```python
from build123d import *

# Parameters (mm, degrees)
SKETCH1_R           = 6.35
BOSS_EXTRUDE1_DEPTH = 3.175
FILLET1_R           = 2
FILLET2_R           = 10
FILLET3_R           = 20


with BuildPart() as part:
    # Sketch1 → Boss-Extrude1 (new, symmetric)
    with BuildSketch(Plane.XY):
        Polygon((75.336239509, 30), (-75.336239509, 30), (-95.474630657, 6), (-95.474630657, -6), (-75.336239509, -30), (75.336239509, -30), (95.474630657, -6), (95.474630657, 6), align=None)
        with BuildLine():
            Line((-88.474630657, -1.3375), (-88.474630657, 1.3375))
            ThreePointArc((-88.474630657, 1.3375), (-88.714791341, 1.656946712), (-88.341203698, 1.798917233))
            ThreePointArc((-88.341203698, 1.798917233), (-82.55, 0), (-88.341203698, -1.798917233))
            ThreePointArc((-88.341203698, -1.798917233), (-88.714791341, -1.656946712), (-88.474630657, -1.3375))
        make_face(mode=Mode.SUBTRACT)
        with Locations((-51.435, 0)):
            Circle(SKETCH1_R, mode=Mode.SUBTRACT)
        with Locations((-17.145, 0)):
            Circle(SKETCH1_R, mode=Mode.SUBTRACT)
        with Locations((17.145, 0)):
            Circle(SKETCH1_R, mode=Mode.SUBTRACT)
        with Locations((51.435, 0)):
            Circle(SKETCH1_R, mode=Mode.SUBTRACT)
        with BuildLine():
            ThreePointArc((88.341203698, 1.798917233), (88.714791341, 1.656946712), (88.474630657, 1.3375))
            Line((88.474630657, 1.3375), (88.474630657, -1.3375))
            ThreePointArc((88.474630657, -1.3375), (88.714791341, -1.656946712), (88.341203698, -1.798917233))
            ThreePointArc((88.341203698, -1.798917233), (82.55, 0), (88.341203698, 1.798917233))
        make_face(mode=Mode.SUBTRACT)
    extrude(amount=BOSS_EXTRUDE1_DEPTH, both=True)

    # Fillet1
    fillet1_edges = [part.edges().sort_by_distance(p)[0] for p in [
        (-88.341203698, 1.798917233, 0),
        (-88.474630657, 1.3375, 0),
        (-88.474630657, -1.3375, 0),
        (-88.341203698, -1.798917233, 0),
        (88.341203698, -1.798917233, 0),
        (88.474630657, -1.3375, 0),
        (88.474630657, 1.3375, 0),
        (88.341203698, 1.798917233, 0),
    ]]
    fillet(fillet1_edges, radius=FILLET1_R)

    # Fillet2
    fillet2_edges = [part.edges().sort_by_distance(p)[0] for p in [
        (95.474630657, 6, 0),
        (95.474630657, -6, 0),
        (-95.474630657, -6, 0),
        (-95.474630657, 6, 0),
    ]]
    fillet(fillet2_edges, radius=FILLET2_R)

    # Fillet3
    fillet3_edges = [part.edges().sort_by_distance(p)[0] for p in [
        (75.336239509, -30, 0),
        (-75.336239509, -30, 0),
        (-75.336239509, 30, 0),
        (75.336239509, 30, 0),
    ]]
    fillet(fillet3_edges, radius=FILLET3_R)


solid = part.part
```
Check sheet for the modelled part. Datum: model origin and axes. Units: mm. Round coordinates to 2 decimals unless told otherwise and drop trailing zeros. Write each loop counter-clockwise with the first axis right and the second up, starting at its lowest first coordinate (ties: lowest second). Pieces come first, ordered by that corner, then holes. Notation, with made-up numbers: (7.25, 51) -> (54.25, 51) arc R33 cw to (54.25, 89) -> close; hole circle Ø10 at (5, 48.25). An arc over 180 degrees is marked (long way). One line per question, with ' | ' between items. Start each with the question number.
1. Sectioned sample at A-A, the plane x = -18. Record the cut outline in (y, z) (3 decimals), then the cut area to 3 significant figures.
2. Depth check by flat-ended pin: pin 1 (1.5 mm diameter, centred on y = 4, z = 1, fed in from -X) (3 decimals); pin 2 (1 mm diameter, centred on y = -4.5, z = 0.5, fed in from +X). Enter the tip coordinate at first touch or a pass-through.
3. Scan lines: line 1 along X through (y, z) = (5, -2.5); line 2 along X through (y, z) = (-7, 1.5); line 3 along Y through (x, z) = (-18.5, -2). Record each from-to range of solid material in increasing order. Write a range as from..to.
4. Release check for a two-part mould opening along Y. For faces 1 (the face through (-95.475, 0, 0)), 2 (the face through (94.855, 5.826, -0.044)), 3 (the face through (-45.38, 1.91, -0.04)) record: +Y half, -Y half, draft (parallel to the pull), parting line (faces both ways), or undercut.
5. Sectioned sample at D-D, the plane x = 79.5. Record the cut outline in (y, z) (3 decimals).
6. Sectioned sample at B-B, the plane z = 2. Count the separate pieces of the cut face and the enclosed holes in it, then the cut area to 3 significant figures.
7. Sectioned sample at C-C, the plane x = -54. Record the cut outline in (y, z) (3 decimals), then the cut area to 3 significant figures.
Taken from the geometry:
1) outline: (-30, -3.175) -> (-6.292, -3.175) -> (-6.292, 3.175) -> (-30, 3.175) -> close; (6.292, -3.175) -> (30, -3.175) -> (30, 3.175) -> (6.292, 3.175) -> close | area: 301 mm^2
2) pin 1: stops at x = -95.435 | pin 2: stops at x = 95.34
3) line 1: x = -95.12..-55.35, -47.52..-21.06, -13.23..13.23, 21.06..47.52, 55.35..95.12 | line 2: x = -94.33..94.33 | line 3: y = -30..-6.2, 6.2..30
4) face 1: draft | face 2: +Y half | face 3: undercut
5) outline: (-24.766, -3.175) -> (24.766, -3.175) -> (24.766, 3.175) -> (-24.766, 3.175) -> close
6) separate pieces: 1 | enclosed holes: 6 | area: 9,870 mm^2
7) outline: (-30, -3.175) -> (-5.809, -3.175) -> (-5.809, 3.175) -> (-30, 3.175) -> close; (5.809, -3.175) -> (30, -3.175) -> (30, 3.175) -> (5.809, 3.175) -> close | area: 307 mm^2
